The model under review builds one solid part; all positions refer to its coordinate system, in mm. Round coordinates to 2 decimals unless told otherwise and drop trailing zeros. Order: outer loops, then holes, each group sorted by start corner. A loop starts at its lowest first (then second) coordinate and runs counter-clockwise, first axis right, second up.
```python
from build123d import *

# Parameters (mm, degrees)
SKETCH_1_R      = 5.05
SKETCH_1_R_2    = 1.55
EXTRUDE_1_DEPTH = 3


with BuildPart() as part:
    # ｽｹｯﾁ1 → ﾎﾞｽ - 押し出し1 (new body)
    with BuildSketch(Plane.XY):
        with BuildLine():
            Line((0, -30), (18, -30))
            Line((18, -30), (18, 30))
            Line((18, 30), (0, 30))
            ThreePointArc((0, 30), (-30, 0), (0, -30))
        make_face()
        Circle(SKETCH_1_R, mode=Mode.SUBTRACT)
        with Locations((15, 27)):
            Circle(SKETCH_1_R_2, mode=Mode.SUBTRACT)
        with Locations((15, -27)):
            Circle(SKETCH_1_R_2, mode=Mode.SUBTRACT)
        with Locations((-16.152077461, 9.846364808)):
            Circle(SKETCH_1_R_2, mode=Mode.SUBTRACT)
        with Locations((2.839602216, 18.702330483)):
            Circle(SKETCH_1_R_2, mode=Mode.SUBTRACT)
    extrude(amount=EXTRUDE_1_DEPTH)


solid = part.part
```
(1) Consider section D-D (x = -1.5). Write out the cut boundary in (y, z).
Data:
outline: (-29.96, 0) - (-4.82, 0) - (-4.82, 3) - (-29.96, 3) - close; (4.82, 0) - (29.96, 0) - (29.96, 3) - (4.82, 3) - close
(2) To check wall thickness, follow probe 1 along Y at (x, z) = (15, 1.5); probe 2 along Y at (x, z) = (3.5, 1.7); probe 3 along Y at (x, z) = (0, 1.9). State the ranges of each line that lie inside material, in increasing order.
Data:
probe 1: y = -30 to -28.55, -25.45 to 25.45, 28.55 to 30
probe 2: y = -30 to -3.64, 3.64 to 17.3, 20.1 to 30
probe 3: y = -30 to -5.05, 5.05 to 30
(3) Consider section C-C (z = 2.1). Write out the cut boundary in (x, y), and give its area (3 significant figures).
Data:
outline: (0, -30) - (18, -30) - (18, 30) - (0, 30) arc R30 ccw to start; hole circle Ø3.1 at (-16.15, 9.85); hole circle Ø10.1 at (0, 0); hole circle Ø3.1 at (2.84, 18.7); hole circle Ø3.1 at (15, -27); hole circle Ø3.1 at (15, 27)
area: 2,380 mm2
(4) Draft analysis for pull direction Y (two halves, no side actions). For faces 1 (the cylindrical face through (2.64, 20.24, 1.48)), 2 (the cylindrical face through (4.817, 1.517, 1.479)), 3 (the flat face through (18, 0, 1)), 4 (the cylindrical face through (-29.993, 0.66, 1.479)), state which applies: pulls with the +Y half, pulls with the -Y half, needs draft (parallel to the pull), parting line crosses it, or undercut.
Data:
face 1: undercut
face 2: undercut
face 3: needs draft
face 4: parting line crosses it
(5) Consider section B-B (y = 0). Write out the cut boundary in (x, z), and give its area (3 significant figures).
Data:
outline: (-30, 0) - (-5.05, 0) - (-5.05, 3) - (-30, 3) - close; (5.05, 0) - (18, 0) - (18, 3) - (5.05, 3) - close
area: 114 mm2
(6) Consider section A-A (x = 15). Write out the cut boundary in (y, z), and give its area (3 significant figures).
Data:
outline: (-30, 0) - (-28.55, 0) - (-28.55, 3) - (-30, 3) - close; (-25.45, 0) - (25.45, 0) - (25.45, 3) - (-25.45, 3) - close; (28.55, 0) - (30, 0) - (30, 3) - (28.55, 3) - close
area: 161 mm2
(7) Insertion check: pin 1 (2.5 mm diameter, centred on x = 15, y = 27, fed in from -Z). The pin has a flat end and moves straight along its axis. Give the tip position at first contact, or say it passes through.
Data:
pin 1: passes through
